Here's how the part is built. I have some questions about the finished solid (model axes, mm). Face numbers are marked on the shaded views. A direction names the side the tool comes from. Give positions to 0.01 mm unless a question says otherwise; leave off trailing zeros. Order: outer loops, then holes, each group sorted by start corner. A loop starts at its lowest first (then second) coordinate and runs counter-clockwise, first axis right, second up. Notation, with made-up numbers: M -10,2.25 L 7,2.25 A11 cw 7,11.25 Z; hole C 71,50 d11. An arc over 180 degrees is marked long. One line per item, written item: value. Start each with the question number.
from build123d import *

# Parameters (mm, degrees)
SKETCH1_W                 = 100
SKETCH1_H                 = 100
BOSS_EXTRUDE1_DEPTH       = 3
SKETCH2_W                 = 100
SKETCH2_H                 = 100
SKETCH2_W_2               = 94
SKETCH2_H_2               = 94
BOSS_EXTRUDE2_DEPTH       = 25
SKETCH5_R                 = 3
CUT_EXTRUDE1_DEPTH        = 146.107718609
SKETCH6_W                 = 12
SKETCH6_H                 = 4
SKETCH6_W_2               = 8
CUT_EXTRUDE3_DEPTH        = 145.166570328
SKETCH7_W                 = 6
SKETCH7_H                 = 20
SKETCH7_W_2               = 20
SKETCH7_H_2               = 6
BOSS_EXTRUDE4_DEPTH       = 25
M4X0_7_TAPPED_HOLE1_D     = 3.3
M4X0_7_TAPPED_HOLE1_DEPTH = 20
M4X0_7_TAPPED_HOLE1_TIP   = 0.991420021
FILLET1_R                 = 1
FILLET2_R                 = 1
FILLET3_R                 = 1
FILLET4_R                 = 1
FILLET5_R                 = 1
FILLET6_R                 = 1
FILLET7_R                 = 1
FILLET8_R                 = 1
FILLET9_R                 = 1
FILLET10_R                = 1
FILLET11_R                = 1
FILLET12_R                = 1
FILLET22_R                = 1
FILLET23_R                = 1
FILLET24_R                = 1
FILLET25_R                = 1
FILLET26_R                = 1
FILLET27_R                = 1
FILLET28_R                = 1
FILLET29_R                = 1
FILLET30_R                = 1
FILLET31_R                = 1
FILLET32_R                = 1
FILLET33_R                = 1
CUT_EXTRUDE5_DEPTH        = 145.166570328


with BuildPart() as part:
    # Sketch1 → Boss-Extrude1 (new body)
    with BuildSketch(Plane.XY):
        with Locations((50, 50)):
            Rectangle(SKETCH1_W, SKETCH1_H)
    extrude(amount=BOSS_EXTRUDE1_DEPTH)

    # Sketch2 → Boss-Extrude2 (add)
    with BuildSketch(Plane.XY.offset(3)):
        with Locations((50, 50)):
            Rectangle(SKETCH2_W, SKETCH2_H)
        with Locations((50, 50)):
            Rectangle(SKETCH2_W_2, SKETCH2_H_2, mode=Mode.SUBTRACT)
    extrude(amount=BOSS_EXTRUDE2_DEPTH)

    # Sketch5 → Cut-Extrude1 (cut, through all)
    with BuildSketch(Plane.XY.offset(32.5)):
        with Locations((8.9, 8.9)):
            Circle(SKETCH5_R)
        with Locations((8.9, 91.1)):
            Circle(SKETCH5_R)
        with Locations((91.1, 91.1)):
            Circle(SKETCH5_R)
        with Locations((91.1, 8.9)):
            Circle(SKETCH5_R)
    extrude(amount=-CUT_EXTRUDE1_DEPTH, mode=Mode.SUBTRACT)

    # Sketch6 → Cut-Extrude3 (cut, through all)
    with BuildSketch(Plane.XZ):
        with Locations((9, 21)):
            Rectangle(SKETCH6_W, SKETCH6_H)
        with Locations((91, 21)):
            Rectangle(SKETCH6_W, SKETCH6_H)
        with Locations((9, 7)):
            Rectangle(SKETCH6_W_2, SKETCH6_H)
        with Locations((91, 7)):
            Rectangle(SKETCH6_W_2, SKETCH6_H)
    extrude(amount=-CUT_EXTRUDE3_DEPTH, mode=Mode.SUBTRACT)

    # Sketch7 → Boss-Extrude4 (add)
    with BuildSketch(Plane.XY.offset(3)):
        with Locations((6, 50)):
            Rectangle(SKETCH7_W, SKETCH7_H)
        with Locations((50, 94)):
            Rectangle(SKETCH7_W_2, SKETCH7_H_2)
        with Locations((94, 50)):
            Rectangle(SKETCH7_W, SKETCH7_H)
        with Locations((50, 6)):
            Rectangle(SKETCH7_W_2, SKETCH7_H_2)
    extrude(amount=BOSS_EXTRUDE4_DEPTH)

    # M4x0.7 Tapped Hole1
    with Locations(Plane.XY.offset(28)):
        with Locations((6, 50), (50, 94), (94, 50), (50, 6)):
            Hole(M4X0_7_TAPPED_HOLE1_D / 2, depth=M4X0_7_TAPPED_HOLE1_DEPTH)
            with Locations((0, 0, -(M4X0_7_TAPPED_HOLE1_DEPTH + M4X0_7_TAPPED_HOLE1_TIP / 2))):  # 118° drill point
                Cone(0, M4X0_7_TAPPED_HOLE1_D / 2, M4X0_7_TAPPED_HOLE1_TIP, mode=Mode.SUBTRACT)

    # Fillet1
    fillet1_edges = [part.edges().sort_by_distance(p)[0] for p in [
        (0, 0, 14),
    ]]
    fillet(fillet1_edges, radius=FILLET1_R)

    # Fillet2
    fillet2_edges = [part.edges().sort_by_distance(p)[0] for p in [
        (100, 0, 14),
    ]]
    fillet(fillet2_edges, radius=FILLET2_R)

    # Fillet3
    fillet3_edges = [part.edges().sort_by_distance(p)[0] for p in [
        (0, 100, 14),
    ]]
    fillet(fillet3_edges, radius=FILLET3_R)

    # Fillet4
    fillet4_edges = [part.edges().sort_by_distance(p)[0] for p in [
        (100, 100, 14),
    ]]
    fillet(fillet4_edges, radius=FILLET4_R)

    # Fillet5
    fillet5_edges = [part.edges().sort_by_distance(p)[0] for p in [
        (40, 3, 15.5),
    ]]
    fillet(fillet5_edges, radius=FILLET5_R)

    # Fillet6
    fillet6_edges = [part.edges().sort_by_distance(p)[0] for p in [
        (60, 3, 15.5),
    ]]
    fillet(fillet6_edges, radius=FILLET6_R)

    # Fillet7
    fillet7_edges = [part.edges().sort_by_distance(p)[0] for p in [
        (97, 40, 15.5),
    ]]
    fillet(fillet7_edges, radius=FILLET7_R)

    # Fillet8
    fillet8_edges = [part.edges().sort_by_distance(p)[0] for p in [
        (97, 60, 15.5),
    ]]
    fillet(fillet8_edges, radius=FILLET8_R)

    # Fillet9
    fillet9_edges = [part.edges().sort_by_distance(p)[0] for p in [
        (3, 60, 15.5),
    ]]
    fillet(fillet9_edges, radius=FILLET9_R)

    # Fillet10
    fillet10_edges = [part.edges().sort_by_distance(p)[0] for p in [
        (3, 40, 15.5),
    ]]
    fillet(fillet10_edges, radius=FILLET10_R)

    # Fillet11
    fillet11_edges = [part.edges().sort_by_distance(p)[0] for p in [
        (40, 97, 15.5),
    ]]
    fillet(fillet11_edges, radius=FILLET11_R)

    # Fillet12
    fillet12_edges = [part.edges().sort_by_distance(p)[0] for p in [
        (60, 97, 15.5),
    ]]
    fillet(fillet12_edges, radius=FILLET12_R)

    # Fillet22
    fillet22_edges = [part.edges().sort_by_distance(p)[0] for p in [
        (60, 9, 15.5),
    ]]
    fillet(fillet22_edges, radius=FILLET22_R)

    # Fillet23
    fillet23_edges = [part.edges().sort_by_distance(p)[0] for p in [
        (40, 9, 15.5),
    ]]
    fillet(fillet23_edges, radius=FILLET23_R)

    # Fillet24
    fillet24_edges = [part.edges().sort_by_distance(p)[0] for p in [
        (91, 60, 15.5),
    ]]
    fillet(fillet24_edges, radius=FILLET24_R)

    # Fillet25
    fillet25_edges = [part.edges().sort_by_distance(p)[0] for p in [
        (91, 40, 15.5),
    ]]
    fillet(fillet25_edges, radius=FILLET25_R)

    # Fillet26
    fillet26_edges = [part.edges().sort_by_distance(p)[0] for p in [
        (9, 60, 15.5),
    ]]
    fillet(fillet26_edges, radius=FILLET26_R)

    # Fillet27
    fillet27_edges = [part.edges().sort_by_distance(p)[0] for p in [
        (9, 40, 15.5),
    ]]
    fillet(fillet27_edges, radius=FILLET27_R)

    # Fillet28
    fillet28_edges = [part.edges().sort_by_distance(p)[0] for p in [
        (60, 91, 15.5),
    ]]
    fillet(fillet28_edges, radius=FILLET28_R)

    # Fillet29
    fillet29_edges = [part.edges().sort_by_distance(p)[0] for p in [
        (40, 91, 15.5),
    ]]
    fillet(fillet29_edges, radius=FILLET29_R)

    # Fillet30
    fillet30_edges = [part.edges().sort_by_distance(p)[0] for p in [
        (21, 3, 3),
        (39.707106781, 3.292893219, 3),
        (60, 6, 3),
        (79, 3, 3),
        (60.292893219, 3.292893219, 3),
        (50, 9, 3),
        (59.707106781, 8.707106781, 3),
        (40, 6, 3),
        (40.292893219, 8.707106781, 3),
    ]]
    fillet(fillet30_edges, radius=FILLET30_R)

    # Fillet31
    fillet31_edges = [part.edges().sort_by_distance(p)[0] for p in [
        (3, 79, 3),
        (3.292893219, 60.292893219, 3),
        (3, 21.5, 3),
        (6, 40, 3),
        (3.292893219, 39.707106781, 3),
        (6, 60, 3),
        (8.707106781, 59.707106781, 3),
        (9, 50, 3),
        (8.707106781, 40.292893219, 3),
        (3, 3.292893219, 3.292893219),
        (3, 3, 11.5),
    ]]
    fillet(fillet31_edges, radius=FILLET31_R)

    # Fillet32
    fillet32_edges = [part.edges().sort_by_distance(p)[0] for p in [
        (79, 97, 3),
        (21.5, 97, 3),
        (40, 94, 3),
        (39.707106781, 96.707106781, 3),
        (60.292893219, 96.707106781, 3),
        (60, 94, 3),
        (59.707106781, 91.292893219, 3),
        (50, 91, 3),
        (40.292893219, 91.292893219, 3),
        (3.292893219, 97, 3.292893219),
        (3, 97, 11.5),
    ]]
    fillet(fillet32_edges, radius=FILLET32_R)

    # Fillet33
    fillet33_edges = [part.edges().sort_by_distance(p)[0] for p in [
        (96.707106781, 39.707106781, 3),
        (97, 78.5, 3),
        (94, 60, 3),
        (96.707106781, 60.292893219, 3),
        (91, 50, 3),
        (91.292893219, 59.707106781, 3),
        (94, 40, 3),
        (91.292893219, 40.292893219, 3),
        (97, 21.5, 3),
        (97, 3.292893219, 3.292893219),
        (97, 97, 11.5),
        (97, 96.707106781, 3.292893219),
        (97, 3, 11.5),
    ]]
    fillet(fillet33_edges, radius=FILLET33_R)

    # Sketch12 → Cut-Extrude5 (cut, through all)
    with BuildSketch(Plane.XZ):
        with BuildLine():
            Line((21, 19), (29, 19))
            ThreePointArc((29, 19), (29.707106781, 19.292893219), (30, 20))
            Line((30, 20), (30, 22))
            ThreePointArc((30, 22), (29.707106781, 22.707106781), (29, 23))
            Line((29, 23), (21, 23))
            ThreePointArc((21, 23), (20.292893219, 22.707106781), (20, 22))
            Line((20, 22), (20, 20))
            ThreePointArc((20, 20), (20.292893219, 19.292893219), (21, 19))
        make_face()
        with BuildLine():
            Line((71, 19), (79, 19))
            ThreePointArc((79, 19), (79.707106781, 19.292893219), (80, 20))
            Line((80, 20), (80, 22))
            ThreePointArc((80, 22), (79.707106781, 22.707106781), (79, 23))
            Line((79, 23), (71, 23))
            ThreePointArc((71, 23), (70.292893219, 22.707106781), (70, 22))
            Line((70, 22), (70, 20))
            ThreePointArc((70, 20), (70.292893219, 19.292893219), (71, 19))
        make_face()
    extrude(amount=-CUT_EXTRUDE5_DEPTH, mode=Mode.SUBTRACT)


solid = part.part
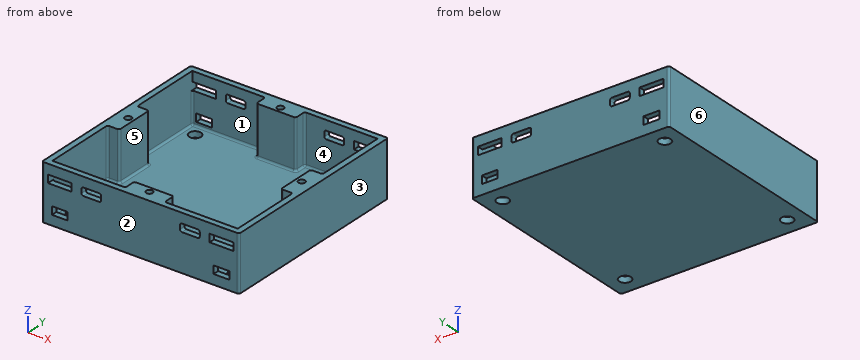
Item 1: I want a section at C-C on z = 17. Count the separate pieces of the cut face and the enclosed holes in it, plus the area to 3 significant figures.
Item 2: Will these pins go through, and if not, where does the flat tip stop? P1, Ø3, axis at x = 25, y = 47.5, coming from the +Z side; P2, Ø2, axis at x = 27, z = 21, coming from the +Y side.
Item 3: Please list where these lines run through material, in increasing order: probe 1 along X at (y, z) = (50, 18.5); probe 2 along Y at (x, z) = (8.9, 1.8). Write a range as [from, to].
Item 4: We'd pull the mould along X, two halves only. Please class the marked faces 1, 2, 3 and 4: +X half, -X half, draft (parallel to the pull), parting line (faces both ways), or undercut.
Item 5: For the marked faces 5 and 6, which set-ups out of +Z, -Z, +X, -X, +Y, -Y let a thin tool reach every point of the face, with its end or its side?
Item 6: I want a section at A-A on x = 34.5. Write out the boundary of the cut face in (y, z).
Answer below:
1. separate pieces: 1
1. enclosed holes: 5
1. area: 1,610 mm²
2. P1: stops at z = 3
2. P2: passes through
3. probe 1: x = [0, 4.35], [7.65, 9], [91, 92.35], [95.65, 100]
3. probe 2: y = [0, 5.9], [11.9, 88.1], [94.1, 100]
4. face 1: undercut
4. face 2: draft
4. face 3: +X half
4. face 4: undercut
5. face 5: +Z
5. face 6: +Z, -Z, -X, +Y, -Y
6. outline: M 0,0 L 100,0 L 100,28 L 97,28 L 97,4 A1 cw 96,3 L 4,3 A1 cw 3,4 L 3,28 L 0,28 Z
